Could you check a few things on this drawing? It's one solid part, dimensions in mm from its lowest x, y, z. Coordinates: 2 decimals unless noted, no trailing zeros. Order: outer loops, then holes, each group sorted by start corner. A loop starts at its lowest first (then second) coordinate and runs counter-clockwise, first axis right, second up. Notation, with made-up numbers: (21, 89) -> (34, 89) arc R15 ccw to (34, 96) -> close; hole circle Ø11 at (46.5, 42). An arc over 180 degrees is marked (long way). Answer as CSV lines item,"result".
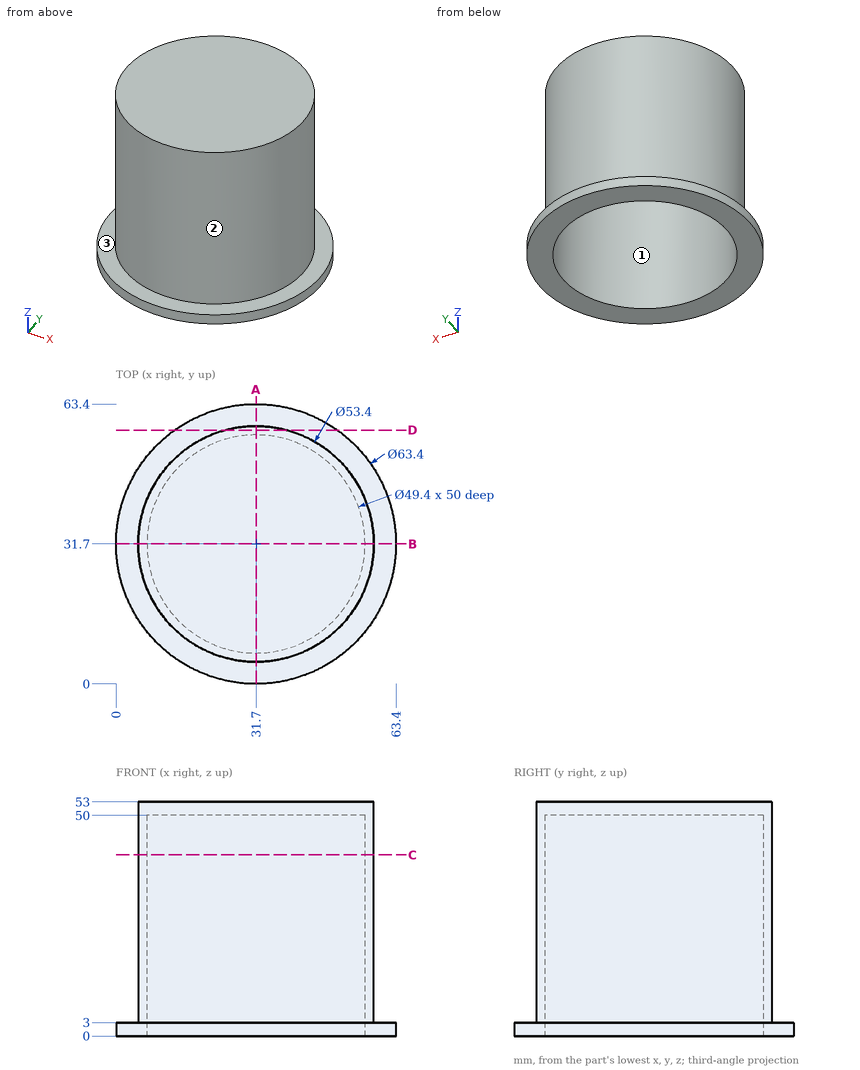
Q1. We'd pull the mould along X, two halves only. Please class the marked faces 1, 2 and 3: pulls with the +X half, pulls with the -X half, needs draft (parallel to the pull), parting line crosses it, or undercut.
Solution:
face 1,"undercut"
face 2,"parting line crosses it"
face 3,"needs draft"
Q2. If I drill on line 1 (X direction, y = 31, z = 15); line 2 (Y direction, x = 31.7, z = 35); line 3 (Z direction, x = 59.5, y = 18.5), over which ranges is the centre line in solid material (lowest first)?
Solution:
line 1,"5.01 to 7.01, 56.39 to 58.39"
line 2,"5 to 7, 56.4 to 58.4"
line 3,"0 to 3"
Q3. Imagine slicing it at C-C (z = 41). List the corners of the cut face in (x, y) for me, and give its area (3 significant figures).
Solution:
outline,"circle Ø53.4 at (31.7, 31.7); hole circle Ø49.4 at (31.7, 31.7)"
area,"323 mm2"
Q4. Imagine slicing it at A-A (x = 31.7). List the corners of the cut face in (y, z) for me, and give its area (3 significant figures).
Solution:
outline,"(0, 0) -> (7, 0) -> (7, 50) -> (56.4, 50) -> (56.4, 0) -> (63.4, 0) -> (63.4, 3) -> (58.4, 3) -> (58.4, 53) -> (5, 53) -> (5, 3) -> (0, 3) -> close"
area,"390 mm2"
Q5. Imagine slicing it at D-D (y = 57.5). List the corners of the cut face in (x, z) for me.
Solution:
outline,"(13.28, 0) -> (50.12, 0) -> (50.12, 3) -> (38.57, 3) -> (38.57, 53) -> (24.83, 53) -> (24.83, 3) -> (13.28, 3) -> close"
Q6. For P1, Ø2, axis at y = 52, z = 6.5, coming from the +X side; P2, Ø1, axis at x = 46.5, z = 33, coming from the -Y side; P3, Ø6, axis at x = 22.5, z = 43.5, coming from the -Y side, each with a flat end and sliding along its axis, tell me the tip position at first contact or that it passes through.
Solution:
P1,"x = 50.15"
P2,"y = 9.15"
P3,"y = 5.73"
